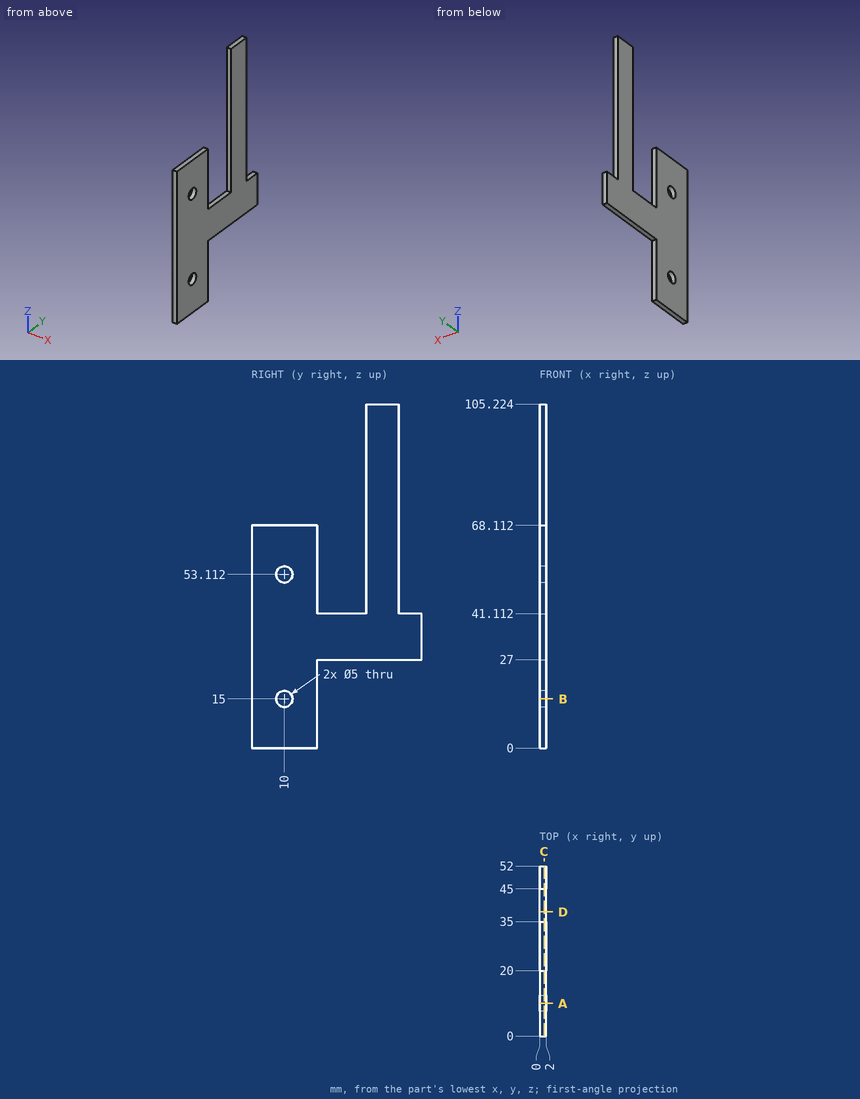
Print and shaded views of the part. All mm, measured from the part's lowest x, y and z. Give positions to 0.01 mm unless a question says otherwise; leave off trailing zeros. Loops run counter-clockwise (first coordinate to the right, second up) from the corner with the lowest first, then second, coordinate; pieces in that order, holes last.
1) Saw through at D-D (y = 38). Write the cut outline in (x, z).
2) Saw through at A-A (y = 10). Write the cut outline in (x, z).
3) Flat gauge pins, fed straight in: pin 1 Ø0.6 at (x, z) = (1, 14) entering from +Y; pin 2 Ø0.6 at (x, y) = (1, 8.5) entering from +Z; pin 3 Ø3 at (y, z) = (10, 15) entering from -X; pin 4 Ø0.6 at (x, z) = (1, 48.5) entering from +Y. Where does each tip first touch, or does it go through?
4) Saw through at C-C (x = 1.35). Write the cut outline in (y, z), plus the area to 3 significant figures.
5) Wall check: line 1 (Z direction, x = 0.6, y = 10); line 2 (Y direction, x = 1.45, z = 42); line 3 (Y direction, x = 0.6, z = 15). Give the ranges that are in metal, low to high.
6) Saw through at B-B (z = 15). Write the cut outline in (x, y), plus the area to 3 significant figures.
Answer block:
1. outline: (0, 27) - (2, 27) - (2, 105.22) - (0, 105.22) - close
2. outline: (0, 0) - (2, 0) - (2, 12.5) - (0, 12.5) - close; (0, 17.5) - (2, 17.5) - (2, 50.61) - (0, 50.61) - close; (0, 55.61) - (2, 55.61) - (2, 68.11) - (0, 68.11) - close
3. pin 1: stops at y = 20
3. pin 2: stops at z = 68.11
3. pin 3: passes through
3. pin 4: stops at y = 45
4. outline: (0, 0) - (20, 0) - (20, 27) - (52, 27) - (52, 41.11) - (45, 41.11) - (45, 105.22) - (35, 105.22) - (35, 41.11) - (20, 41.11) - (20, 68.11) - (0, 68.11) - close; hole circle Ø5 at (10, 15); hole circle Ø5 at (10, 53.11)
4. area: 2,420 mm2
5. line 1: z = 0 to 12.5, 17.5 to 50.61, 55.61 to 68.11
5. line 2: y = 0 to 20, 35 to 45
5. line 3: y = 0 to 7.5, 12.5 to 20
6. outline: (0, 0) - (2, 0) - (2, 7.5) - (0, 7.5) - close; (0, 12.5) - (2, 12.5) - (2, 20) - (0, 20) - close
6. area: 30.0 mm2
